Autodesk Inventor part; units mm, degrees
ref_plane "YZ Plane" through (0, 0, 0) normal (1, 0, 0) x (0, 1, 0)
ref_plane "XZ Plane" through (0, 0, 0) normal (0, 1, 0) x (-1, 0, 0)
ref_plane "XY Plane" through (0, 0, 0) normal (0, 0, 1) x (1, 0, 0)
sketch "Sketch1" plane through (0, 0, 0) normal (0, 0, 1) x (1, 0, 0)
  arc A0 (-1.6262, -4.5044) -> (-3.8713, -5.4343) centre (-1.6262, -7.6794) ccw
  line L0 (1.6262, -4.5044) -> (-1.6262, -4.5044)
  arc A1 (3.8713, -5.4343) -> (1.6262, -4.5044) centre (1.6262, -7.6794) ccw
  line L1 (7.1551, -8.7181) -> (3.8713, -5.4343)
  arc A2 (6.3985, -10.4902) -> (7.1551, -8.7181) centre (6.3689, -9.43) ccw
  line L2 (-6.4049, -10.4902) -> (6.3985, -10.4902)
  arc A3 (-7.1552, -8.7184) -> (-6.4049, -10.4902) centre (-6.369, -9.4302) ccw
  line L3 (-3.8713, -5.4343) -> (-7.1552, -8.7184)
  circle A4 centre (0, 0) radius 2.6035
  arc A5 (-4.5044, 1.6262) -> (-5.4343, 3.8713) centre (-7.6794, 1.6262) ccw
  line L4 (-4.5044, -1.6262) -> (-4.5044, 1.6262)
  arc A6 (-5.4343, -3.8713) -> (-4.5044, -1.6262) centre (-7.6794, -1.6262) ccw
  line L5 (-8.7181, -7.1551) -> (-5.4343, -3.8713)
  arc A7 (-10.4902, -6.3985) -> (-8.7181, -7.1551) centre (-9.43, -6.3689) ccw
  line L6 (-10.4902, 6.4049) -> (-10.4902, -6.3985)
  arc A8 (-8.7184, 7.1552) -> (-10.4902, 6.4049) centre (-9.4302, 6.369) ccw
  line L7 (-5.4343, 3.8713) -> (-8.7184, 7.1552)
  arc A9 (8.7184, -7.1552) -> (10.4902, -6.4049) centre (9.4302, -6.369) ccw
  line L8 (5.4343, -3.8713) -> (8.7184, -7.1552)
  arc A10 (4.5044, -1.6262) -> (5.4343, -3.8713) centre (7.6794, -1.6262) ccw
  line L9 (4.5044, 1.6262) -> (4.5044, -1.6262)
  arc A11 (5.4343, 3.8713) -> (4.5044, 1.6262) centre (7.6794, 1.6262) ccw
  line L10 (8.7181, 7.1551) -> (5.4343, 3.8713)
  arc A12 (10.4902, 6.3985) -> (8.7181, 7.1551) centre (9.43, 6.3689) ccw
  line L11 (10.4902, -6.4049) -> (10.4902, 6.3985)
  arc A13 (12.7, -9.5504) -> (12.7, -10.5664) centre (12.7, -10.0584) ccw
  line L12 (12.7, -9.5504) -> (12.7, -6.604)
  arc A14 (12.7, -5.588) -> (12.7, -6.604) centre (12.7, -6.096) ccw
  line L13 (12.7, -5.588) -> (12.7, 5.588)
  arc A15 (12.7, 6.604) -> (12.7, 5.588) centre (12.7, 6.096) ccw
  line L14 (12.7, 6.604) -> (12.7, 9.5504)
  arc A16 (12.7, 10.5664) -> (12.7, 9.5504) centre (12.7, 10.0584) ccw
  line L15 (12.7, 10.5664) -> (12.7, 10.5918)
  arc A17 (12.7, 10.5918) -> (10.5918, 12.7) centre (10.5918, 10.5918) ccw
  line L16 (10.5918, 12.7) -> (10.5664, 12.7)
  arc A18 (9.5504, 12.7) -> (10.5664, 12.7) centre (10.0584, 12.7) ccw
  line L17 (9.5504, 12.7) -> (6.604, 12.7)
  arc A19 (5.588, 12.7) -> (6.604, 12.7) centre (6.096, 12.7) ccw
  line L18 (5.588, 12.7) -> (4.3561, 12.7)
  arc A20 (4.3561, 12.7) -> (4.3561, 10.4902) centre (4.3561, 11.5951) ccw
  line L19 (4.3561, 10.4902) -> (6.4049, 10.4902)
  arc A21 (7.1552, 8.7184) -> (6.4049, 10.4902) centre (6.369, 9.4302) ccw
  line L20 (7.1552, 8.7184) -> (3.8713, 5.4343)
  arc A22 (1.6262, 4.5044) -> (3.8713, 5.4343) centre (1.6262, 7.6794) ccw
  line L21 (1.6262, 4.5044) -> (-1.6262, 4.5044)
  arc A23 (-3.8713, 5.4343) -> (-1.6262, 4.5044) centre (-1.6262, 7.6794) ccw
  line L22 (-3.8713, 5.4343) -> (-7.1551, 8.7181)
  arc A24 (-6.3985, 10.4902) -> (-7.1551, 8.7181) centre (-6.3689, 9.43) ccw
  line L23 (-6.3985, 10.4902) -> (-4.3561, 10.4902)
  arc A25 (-4.3561, 10.4902) -> (-4.3561, 12.7) centre (-4.3561, 11.5951) ccw
  line L24 (-4.3561, 12.7) -> (-5.588, 12.7)
  arc A26 (-6.604, 12.7) -> (-5.588, 12.7) centre (-6.096, 12.7) ccw
  line L25 (-6.604, 12.7) -> (-9.5504, 12.7)
  arc A27 (-10.5664, 12.7) -> (-9.5504, 12.7) centre (-10.0584, 12.7) ccw
  line L26 (-10.5664, 12.7) -> (-10.5918, 12.7)
  arc A28 (-10.5918, 12.7) -> (-12.7, 10.5918) centre (-10.5918, 10.5918) ccw
  line L27 (-12.7, 10.5918) -> (-12.7, 10.5664)
  arc A29 (-12.7, 9.5504) -> (-12.7, 10.5664) centre (-12.7, 10.0584) ccw
  line L28 (-12.7, 9.5504) -> (-12.7, 6.604)
  arc A30 (-12.7, 5.588) -> (-12.7, 6.604) centre (-12.7, 6.096) ccw
  line L29 (-12.7, 5.588) -> (-12.7, -5.588)
  arc A31 (-12.7, -6.604) -> (-12.7, -5.588) centre (-12.7, -6.096) ccw
  line L30 (-12.7, -6.604) -> (-12.7, -9.5504)
  arc A32 (-12.7, -10.5664) -> (-12.7, -9.5504) centre (-12.7, -10.0584) ccw
  line L31 (-12.7, -10.5664) -> (-12.7, -10.5918)
  arc A33 (-12.7, -10.5918) -> (-10.5918, -12.7) centre (-10.5918, -10.5918) ccw
  line L32 (-10.5918, -12.7) -> (-10.5664, -12.7)
  arc A34 (-9.5504, -12.7) -> (-10.5664, -12.7) centre (-10.0584, -12.7) ccw
  line L33 (-9.5504, -12.7) -> (-6.604, -12.7)
  arc A35 (-5.588, -12.7) -> (-6.604, -12.7) centre (-6.096, -12.7) ccw
  line L34 (-5.588, -12.7) -> (5.588, -12.7)
  arc A36 (6.604, -12.7) -> (5.588, -12.7) centre (6.096, -12.7) ccw
  line L35 (6.604, -12.7) -> (9.5504, -12.7)
  arc A37 (10.5664, -12.7) -> (9.5504, -12.7) centre (10.0584, -12.7) ccw
  line L36 (10.5664, -12.7) -> (10.5918, -12.7)
  arc A38 (10.5918, -12.7) -> (12.7, -10.5918) centre (10.5918, -10.5918) ccw
  line L37 (12.7, -10.5918) -> (12.7, -10.5664)
extrude "Extrusion1" add sketch "Sketch1" against normal blind 304.8
properties part number "1001"
Part model, mm, in its own coordinate system. A direction names the side the tool comes from. Coordinates: 2 decimals unless noted, no trailing zeros.
(1) Slice it at A-A, the plane z = -215. State how many separate pieces and enclosed holes the cut face has, and give its area (3 significant figures).
Check sheet entries:
separate pieces: 1
enclosed holes: 4
area: 327 mm2
(2) Probe L1, parallel to Y at x = 4, z = -59.5; L2, parallel to Y at x = 0, z = -138; L3, parallel to X at y = -0.5, z = -66. List the from-to ranges inside material, lowest first.
Check sheet entries:
L1: y = -12.7 to -10.49, -5.56 to 5.56, 10.55 to 12.64
L2: y = -12.7 to -10.49, -4.5 to -2.6, 2.6 to 4.5
L3: x = -12.7 to -10.49, -4.5 to -2.56, 2.56 to 4.5, 10.49 to 12.7
(3) Pull direction Y, two halves, no side cores. Call faces 1 (the face through (10.49, 0, -150)), 2 (the face through (0, -12.7, -150)), 3 (the face through (0, -3, 0)): pulls with the +Y half, pulls with the -Y half, needs draft (parallel to the pull), parting line crosses it, or undercut.
Check sheet entries:
face 1: undercut
face 2: pulls with the -Y half
face 3: needs draft
(4) Pin check, flat tips, straight feed: pin 1 Ø5 at (x, z) = (1.5, -240.5) entering from +Y; pin 2 Ø8 at (x, y) = (-9, -7.5) entering from +Z; pin 3 Ø1 at (x, z) = (0.5, -114.5) entering from +Y; pin 4 Ø1 at (x, y) = (-8.5, 3) entering from +Z. Stop position of each tip, or through.
Check sheet entries:
pin 1: stops at y = 12.64
pin 2: stops at z = 0
pin 3: stops at y = 4.5
pin 4: passes through
(5) Tool access for faces 4 (the face through (-12.7, 0, -150)), 5 (the face through (-10.49, 0, -150)): list every direction of +Z, -Z, +X, -X, +Y, -Y with a clear straight run to the whole face (end or side of a thin tool).
Check sheet entries:
face 4: +Z, -Z, -X, +Y, -Y
face 5: +Z, -Z
